The listing builds one solid part. Answer for the finished solid, in the listing's coordinates (mm). A direction names the side the tool comes from. Coordinates: 2 decimals unless noted, no trailing zeros. Order: outer loops, then holes, each group sorted by start corner. A loop starts at its lowest first (then second) coordinate and runs counter-clockwise, first axis right, second up.
```python
from build123d import *

# Parameters (mm, degrees)
F0_W     = 30
F0_H     = 20
F0_R     = 5
F1_DEPTH = 10
F2_W     = 2
F2_H     = 20
F3_DEPTH = 4
F5_DEPTH = 20
F6_R     = 2.5
F7_DEPTH = 6


with BuildPart() as f1:
    # F0 (on Front) → F1 (new body)
    with BuildSketch(Plane.XZ):
        Rectangle(F0_W, F0_H)
        Circle(F0_R, mode=Mode.SUBTRACT)
    extrude(amount=F1_DEPTH)

    # F2 (on face) → F3 (cut)
    with BuildSketch(Plane.XZ.offset(10)):
        with Locations((-10, 0)):
            Rectangle(F2_W, F2_H)
        with BuildLine():
            Line((2.5, 10), (-2.5, 10))
            Line((-2.5, 10), (-2.5, 4.330127))
            ThreePointArc((-2.5, 4.330127), (0, 5), (2.5, 4.330127))
            Line((2.5, 4.330127), (2.5, 10))
        make_face()
        with BuildLine():
            Line((-2.5, -4.330127), (-2.5, -10))
            Line((-2.5, -10), (2.5, -10))
            Line((2.5, -10), (2.5, -4.330127))
            ThreePointArc((2.5, -4.330127), (0, -5), (-2.5, -4.330127))
        make_face()
    extrude(amount=-F3_DEPTH, mode=Mode.SUBTRACT)

    # F4 (on face) → F5 (cut, through all)
    with BuildSketch(Plane(origin=(0, 0, -10), x_dir=(1, 0, 0), z_dir=(0, 0, -1))):
        Polygon((10, 10), (6, 10), (3.690599, 6), (12.309401, 6), align=None)
    extrude(amount=-F5_DEPTH, mode=Mode.SUBTRACT)

    # F6 (on face) → F7 (join)
    with BuildSketch(Plane.YZ.offset(15)):
        with Locations((-5, 0)):
            Circle(F6_R)
    extrude(amount=F7_DEPTH)


solid = f1.part
```
1) A cutting plane is placed at C-C, the plane y = -5. Write down the section's boundary in (x, z), plus the area to 3 significant figures.
2) For faces 1 (the flat face through (2.5, -8, -7)), 2 (the flat face through (15, -3.8, -2.4)), 3 (the flat face through (21, -5, 0)), determine the directions among +Z, -Z, +X, -X, +Y, -Y from which every point of the face is accessible in a straight line to the end or side of a thin tool.
3) A cutting plane is placed at B-B, the plane z = -0.5. Write down the section's boundary in (x, y), plus the area to 3 significant figures.
4) A cutting plane is placed at A-A, the plane x = 0. Write down the section's boundary in (y, z).
5) The mould has two halves that part along Z. Classify faces 4 (the cylindrical face through (-4, -4, 3)), 5 (the flat face through (-2.5, -8, 7)), 6 (the cylindrical face through (17.958, -2.615, 0.751)): released by +Z, released by -Z, zero draft, split by the parting line, or undercut.
6) Each of these flat-tipped pins is pushed along its axis until it touches: P1, Ø2.5, axis at x = -1, z = -6, coming from the -Y side; P2, Ø3, axis at x = 1.5, z = 0.5, coming from the -Y side; P3, Ø4.5, axis at y = -8, z = 7, coming from the +X side. Where does it stop, or does it pass through?
7) Straight lines are drawn through the part: probe 1 along X at (y, z) = (-9.25, 8.5); probe 2 along Z at (x, y) = (0, -4); probe 3 along X at (y, z) = (-7, -6.5). For each, find the intervals that lie inside material, in ascending order.
8) A cutting plane is placed at D-D, the plane x = 17.5. Write down the section's boundary in (y, z), plus the area to 3 significant figures.
Working result:
1. outline: (-15, -10) - (15, -10) - (15, -2.5) - (21, -2.5) - (21, 2.5) - (15, 2.5) - (15, 10) - (-15, 10) - close; hole circle Ø10 at (0, 0)
1. area: 551 mm2
2. face 1: +Z, -Z, -Y
2. face 2: +X
2. face 3: +Z, -Z, +X, +Y, -Y
3. outline: (-15, -10) - (-11, -10) - (-11, -6) - (-9, -6) - (-9, -10) - (-4.97, -10) - (-4.97, 0) - (-15, 0) - close; (4.97, -10) - (6, -10) - (4.97, -8.22) - close; (4.97, -6) - (12.31, -6) - (10, -10) - (15, -10) - (15, -7.45) - (21, -7.45) - (21, -2.55) - (15, -2.55) - (15, 0) - (4.97, 0) - close
3. area: 198 mm2
4. outline: (-6, -10) - (0, -10) - (0, -5) - (-6, -5) - close; (-6, 5) - (0, 5) - (0, 10) - (-6, 10) - close
5. face 4: undercut
5. face 5: zero draft
5. face 6: split by the parting line
6. P1: stops at y = -6
6. P2: passes through
6. P3: stops at x = 15
7. probe 1: x = -15 to -11, -9 to -2.5, 2.5 to 5.57, 10.43 to 15
7. probe 2: z = -10 to -5, 5 to 10
7. probe 3: x = -15 to -11, -9 to -2.5, 2.5 to 4.27, 11.73 to 15
8. outline: circle Ø5 at (-5, 0)
8. area: 19.6 mm2
